Here's how the part is built. I have some questions about the finished solid (model axes, mm). A direction names the side the tool comes from. Give positions to 0.01 mm unless a question says otherwise; leave off trailing zeros. Write each loop counter-clockwise with the first axis right and the second up, starting at its lowest first coordinate (ties: lowest second). Pieces come first, ordered by that corner, then holes. Notation, with made-up numbers: (4, -8) -> (29, -8) arc R19 ccw to (29, 14) -> close; hole circle Ø6 at (-8.5, -6). An arc over 180 degrees is marked (long way). Use CSV: the item, a comma, the result in double quotes. Start each with the question number.
(1) Suppose I cut it at A-A on x = 0. List the corners of the cut face in (y, z) for me (3 decimals).
(2) Suppose I cut it at D-D on y = 35. List the corners of the cut face in (x, z) for me.
(3) Suppose I cut it at C-C on y = 87.5. List the corners of the cut face in (x, z) for me.
(4) If we mould it in two halves opening along X, with no side actions, what happens to faces 4 (the flat face through (0, 25.4, 0)), 5 (the cylindrical face through (1.38, 51.65, 6.2)), 6 (the flat face through (-3, 0, 0))? For each: pulls with the +X half, pulls with the -X half, needs draft (parallel to the pull), parting line crosses it, or undercut.
(5) Which directions (+Z, -Z, +X, -X, +Y, -Y) give clear straight access to the entire face, cutting with the end or side of a thin tool? Please do faces 1 (the flat face through (-3, 104.775, 0)), 2 (the cylindrical face through (-0.748, 12.878, -2.374)), 3 (the flat face through (0, 79.375, 0)).
(6) I need wall thicknesses on L1, parallel to Z at x = 0, y = 85; L2, parallel to X at y = 81, z = -1; L3, parallel to X at y = 40.5, z = -3. Which ranges of each line are inside material? Lowest first, please. Write a range as [from, to].
(7) Suppose I cut it at B-B on z = 0. List the corners of the cut face in (x, y) for me (3 decimals).
(8) For pin 1 Ø3 at (x, z) = (0, 0) entering from +Y (3 decimals); pin 2 Ø5 at (y, z) = (17, 3) entering from +X; pin 3 Ø2 at (x, y) = (-1.5, 20) entering from -Z, each with a flat end and sliding along its axis, tell me the tip position at first contact or that it passes through.
Autodesk Inventor part; units mm, degrees
ref_plane "YZ Plane" through (0, 0, 0) normal (1, 0, 0) x (0, 1, 0)
ref_plane "XZ Plane" through (0, 0, 0) normal (0, 1, 0) x (-1, 0, 0)
ref_plane "XY Plane" through (0, 0, 0) normal (0, 0, 1) x (1, 0, 0)
sketch "Sketch1" plane through (0, 0, 0) normal (0, 1, 0) x (-1, 0, 0)
  circle A0 centre (0, 0) radius 6.35
  dimension "d0" = 12.7
extrude "Extrusion1" add sketch "Sketch1" along normal blind 104.775
sketch "Sketch2" plane through (0, 0, 0) normal (0, -1, 0) x (1, 0, 0)
  point P0 (0, 0)
  point P1 (0, 0)
hole "Hole1" at (0, 0, 0) direction (0, 1, 0) diameter 4.9784 depth 25.4
sketch "Sketch3" plane through (0, 104.775, 0) normal (0, 1, 0) x (1, 0, 0)
  point P0 (0, 0)
  point P1 (0, 0)
hole "Hole2" at (0, 104.775, 0) direction (0, -1, 0) diameter 4.9784 depth 25.4
properties part number "SHOT_020_Spacer7" material "Aluminum 6061"
Geometry says:
1,outline,"(0, -6.35) -> (104.775, -6.35) -> (104.775, -2.489) -> (79.375, -2.489) -> (79.375, 2.489) -> (104.775, 2.489) -> (104.775, 6.35) -> (0, 6.35) -> (0, 2.489) -> (25.4, 2.489) -> (25.4, -2.489) -> (0, -2.489) -> close"
2,outline,"circle Ø12.7 at (0, 0)"
3,outline,"circle Ø12.7 at (0, 0); hole circle Ø4.98 at (0, 0)"
4,face 4,"undercut"
4,face 5,"parting line crosses it"
4,face 6,"needs draft"
5,face 1,"+Z, -Z, +X, -X, +Y"
5,face 2,"-Y"
5,face 3,"+Y"
6,L1,"[-6.35, -2.49], [2.49, 6.35]"
6,L2,"[-6.27, -2.28], [2.28, 6.27]"
6,L3,"[-5.6, 5.6]"
7,outline,"(-6.35, 0) -> (-2.489, 0) -> (-2.489, 25.4) -> (2.489, 25.4) -> (2.489, 0) -> (6.35, 0) -> (6.35, 104.775) -> (2.489, 104.775) -> (2.489, 79.375) -> (-2.489, 79.375) -> (-2.489, 104.775) -> (-6.35, 104.775) -> close"
8,pin 1,"y = 79.375"
8,pin 2,"x = 6.33"
8,pin 3,"z = -6.33"
